The model under review builds one solid part; all positions refer to its coordinate system, in mm. Coordinates: 2 decimals unless noted, no trailing zeros. Write each loop counter-clockwise with the first axis right and the second up, starting at its lowest first coordinate (ties: lowest second). Pieces come first, ordered by that corner, then holes. Notation, with made-up numbers: (27, 46) - (60, 46) arc R26 ccw to (60, 64) - close; hole circle Ø2 at (62.5, -37.5). An arc over 180 degrees is marked (long way). Return JSON: item names as keys, results as strings. Group by question number.
(1) We need section B-B on x = -1. State the section outline as (y, z) points, then the cut area to 3 significant figures.
(2) We need section D-D on x = -13.5. State the section outline as (y, z) points, then the cut area to 3 significant figures.
(3) We need section C-C on y = 1. Give the number of separate pieces and of enclosed holes in the cut face, then the cut area to 3 significant figures.
(4) For pin 1 Ø0.8 at (y, z) = (1, 22) entering from +X; pin 2 Ø4.5 at (x, z) = (0, -25.5) entering from +Y; pin 3 Ø0.8 at (y, z) = (1, 5) entering from +X; pin 4 Ø3.5 at (x, z) = (-9.5, -25.5) entering from +Y, all flat-tipped, find the tip position at first contact; note any pin that passes through.
(5) We need section A-A on z = -25.5. State the section outline as (x, y) points.
(6) To check wall thickness, follow L1, parallel to X at y = 0.5, z = -25.5; L2, parallel to X at y = 0.65, z = 13.5; L3, parallel to Z at x = -11, y = 1.1. State the ranges of each line that lie inside material, in increasing order. Write a range as from..to.
```python
from build123d import *

# Parameters (mm, degrees)
SKETCH_1_R      = 2
SKETCH_1_R_2    = 1.5
EXTRUDE_1_DEPTH = 1.5


with BuildPart() as part:
    # 草图1 → 凸台-拉伸1 (new body)
    with BuildSketch(Plane(origin=(0, 0, 0), x_dir=(1, 0, 0), z_dir=(0, 1, 0))):
        Polygon((19.989240701, 17.010759299), (19.989240701, 34.032277896), (15.994131292, 38.027387305), (15.994131292, 51.001956236), (12.496087528, 54.5), (-12.496087528, 54.5), (-15.994131292, 51.001956236), (-15.994131292, 38.027387305), (-19.989240701, 34.032277896), (-19.989240701, 17.010759299), (-16.021518597, 13.043037194), (-16.021518597, 3.543037194), (-12.510759299, 0.032277896), (-12.510759299, -10.032277896), (-16.021518597, -13.543037194), (-16.021518597, -43.5), (-12.521518597, -47), (12.521518597, -47), (16.021518597, -43.5), (16.021518597, -13.543037194), (12.510759299, -10.032277896), (12.510759299, 0.032277896), (16.021518597, 3.543037194), (16.021518597, 13.043037194), align=None)
        with Locations(Location((0, 25.5, 0), (0, 0, 270))):
            Circle(SKETCH_1_R, mode=Mode.SUBTRACT)
        with Locations(Location((9.5, 25.5, 0), (0, 0, 270))):
            Circle(SKETCH_1_R, mode=Mode.SUBTRACT)
        with Locations(Location((11, 3.5, 0), (0, 0, 270))):
            Circle(SKETCH_1_R_2, mode=Mode.SUBTRACT)
        with Locations(Location((11, 47.5, 0), (0, 0, 270))):
            Circle(SKETCH_1_R_2, mode=Mode.SUBTRACT)
        with Locations(Location((-11, 47.5, 0), (0, 0, 90))):
            Circle(SKETCH_1_R_2, mode=Mode.SUBTRACT)
        with Locations(Location((-11, 3.5, 0), (0, 0, 90))):
            Circle(SKETCH_1_R_2, mode=Mode.SUBTRACT)
        with Locations(Location((11, -13.5, 0), (0, 0, 270))):
            Circle(SKETCH_1_R_2, mode=Mode.SUBTRACT)
        with Locations(Location((11, -43.5, 0), (0, 0, 270))):
            Circle(SKETCH_1_R_2, mode=Mode.SUBTRACT)
        with Locations(Location((-11, -13.5, 0), (0, 0, 90))):
            Circle(SKETCH_1_R_2, mode=Mode.SUBTRACT)
        with Locations(Location((-11, -43.5, 0), (0, 0, 90))):
            Circle(SKETCH_1_R_2, mode=Mode.SUBTRACT)
        with Locations(Location((0, 16, 0), (0, 0, 270))):
            Circle(SKETCH_1_R, mode=Mode.SUBTRACT)
        with Locations(Location((-9.5, 25.5, 0), (0, 0, 270))):
            Circle(SKETCH_1_R, mode=Mode.SUBTRACT)
        with Locations(Location((0, 35, 0), (0, 0, 270))):
            Circle(SKETCH_1_R, mode=Mode.SUBTRACT)
    extrude(amount=EXTRUDE_1_DEPTH)


solid = part.part
```
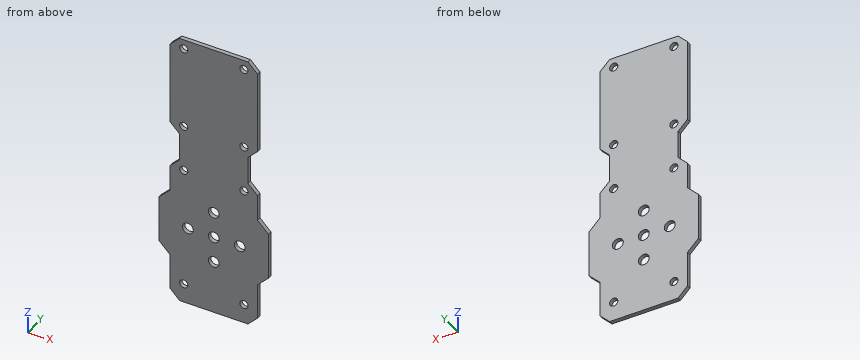
Ans:
{
 "1": {"outline": "(0, -54.5) - (1.5, -54.5) - (1.5, -36.73) - (0, -36.73) - close; (0, -33.27) - (1.5, -33.27) - (1.5, -27.23) - (0, -27.23) - close; (0, -23.77) - (1.5, -23.77) - (1.5, -17.73) - (0, -17.73) - close; (0, -14.27) - (1.5, -14.27) - (1.5, 47) - (0, 47) - close", "area": "137 mm²"},
 "2": {"outline": "(0, -53.5) - (1.5, -53.5) - (1.5, -1.02) - (0, -1.02) - close; (0, 11.02) - (1.5, 11.02) - (1.5, 46.02) - (0, 46.02) - close", "area": "131 mm²"},
 "3": {"separate pieces": "1", "enclosed holes": "13", "area": "3,180 mm²"},
 "4": {"pin 1": "x = 16.02", "pin 2": "y = 1.5", "pin 3": "x = 12.51", "pin 4": "through"},
 "5": {"outline": "(-19.99, 0) - (-11.5, 0) - (-11.5, 1.5) - (-19.99, 1.5) - close; (-7.5, 0) - (-2, 0) - (-2, 1.5) - (-7.5, 1.5) - close; (2, 0) - (7.5, 0) - (7.5, 1.5) - (2, 1.5) - close; (11.5, 0) - (19.99, 0) - (19.99, 1.5) - (11.5, 1.5) - close"},
 "6": {"L1": "-19.99..-11.5, -7.5..-2, 2..7.5, 11.5..19.99", "L2": "-15.98..-12.5, -9.5..9.5, 12.5..15.98", "L3": "-54.5..-49, -46..-26.82, -24.18..-5, -2..12, 15..42, 45..47"}
}
